Can you work these out from the model? Positions are in its coordinate system, mm. A direction names the side the tool comes from. Coordinates: 2 decimals unless noted, no trailing zeros. Order: outer loops, then holes, each group sorted by start corner. A loop starts at its lowest first (then second) coordinate and runs counter-clockwise, first axis right, second up. Notation, with made-up numbers: (50.5, 0.25) -> (57.5, 0.25) arc R25 cw to (57.5, 27.25) -> close; hole circle Ø5 at (78, 8.5). An arc over 180 degrees is marked (long way). Answer in a Markdown table with one row per item.
```python
from build123d import *

# Parameters (mm, degrees)
ESQUISSE1_R                  = 18.5
BOSS_EXTRU_1_DEPTH           = 30.7
ESQUISSE2_R                  = 5
BOSS_EXTRU_2_DEPTH           = 6
ESQUISSE3_R                  = 3
BOSS_EXTRU_3_DEPTH           = 16
ENL_V_MAT_EXTRU_2_DEPTH      = 59.836978168
ENL_V_MAT_EXTRU_2_DEPTH_BACK = 16


with BuildPart() as part:
    # Esquisse1 → Boss.-Extru.1 (new body)
    with BuildSketch(Plane.XY):
        Circle(ESQUISSE1_R)
    extrude(amount=BOSS_EXTRU_1_DEPTH)

    # Esquisse2 → Boss.-Extru.2 (add)
    with BuildSketch(Plane(origin=(0, 0, 0), x_dir=(-1, 0, 0), z_dir=(0, 0, -1))):
        Circle(ESQUISSE2_R)
    extrude(amount=BOSS_EXTRU_2_DEPTH)

    # Esquisse3 → Boss.-Extru.3 (add)
    with BuildSketch(Plane(origin=(0, 0, -6), x_dir=(-1, 0, 0), z_dir=(0, 0, -1))):
        Circle(ESQUISSE3_R)
    extrude(amount=BOSS_EXTRU_3_DEPTH)

    # Esquisse4 → Enlèv. mat.-Extru.2 (cut, two sides: drawn at the far end of the back side and taken through both)
    with BuildSketch(Plane(origin=(0, 0, -22), x_dir=(-1, 0, 0), z_dir=(0, 0, -1)).offset(-ENL_V_MAT_EXTRU_2_DEPTH_BACK)):
        Polygon((-70.071777045, 2.4), (-1.8, 2.4), (1.8, 2.4), (70.071777045, 2.4), (70.071777045, 138.94355409), (-70.071777045, 138.94355409), align=None)
    extrude(amount=ENL_V_MAT_EXTRU_2_DEPTH + ENL_V_MAT_EXTRU_2_DEPTH_BACK, mode=Mode.SUBTRACT)


solid = part.part
```
(1) Suppose I cut it at A-A (y = 0). Please give me the cut outline in (x, z).
Response values:
| item | result |
|---|---|
| outline | (-18.5, 0) -> (-5, 0) -> (-5, -6) -> (-3, -6) -> (-3, -22) -> (3, -22) -> (3, -6) -> (5, -6) -> (5, 0) -> (18.5, 0) -> (18.5, 30.7) -> (-18.5, 30.7) -> close |
(2) Suppose I cut it at D-D (z = -4). Please give me the cut outline in (x, y).
Response values:
| item | result |
|---|---|
| outline | circle Ø10 at (0, 0) |
(3) Suppose I cut it at C-C (z = -11). Please give me the cut outline in (x, y), and give its area (3 significant figures).
Response values:
| item | result |
|---|---|
| outline | (-1.8, 2.4) arc R3 ccw (long way) to (1.8, 2.4) -> close |
| area | 26.8 mm2 |
(4) Suppose I cut it at B-B (x = 0). Please give me the cut outline in (y, z), and give its area (3 significant figures).
Response values:
| item | result |
|---|---|
| outline | (-18.5, 0) -> (-5, 0) -> (-5, -6) -> (-3, -6) -> (-3, -22) -> (2.4, -22) -> (2.4, -6) -> (5, -6) -> (5, 0) -> (18.5, 0) -> (18.5, 30.7) -> (-18.5, 30.7) -> close |
| area | 1,280 mm2 |
(5) Will these pins go through, and if not, where does the flat tip stop? pin 1 Ø2 at (x, z) = (13, 25) entering from +Y; pin 2 Ø1.8 at (x, z) = (-0.5, -15) entering from +Y; pin 3 Ø12 at (y, z) = (-7.5, 5.5) entering from +X.
Response values:
| item | result |
|---|---|
| pin 1 | y = 14.08 |
| pin 2 | y = 2.4 |
| pin 3 | x = 18.44 |
(6) On a 3-axis mill with a long thin cutter (end or side, diameter ignored), from which of +Z, -Z, +X, -X, +Y, -Y can I reach the whole of each face in a straight line? I mean faces 1 (the cylindrical face through (0, -3, -14)), 2 (the flat face through (0, 2.4, -14)), 3 (the flat face through (0, 0, -22)). Say none if no direction works.
Response values:
| item | result |
|---|---|
| face 1 | -Z |
| face 2 | -Z, +X, -X, +Y |
| face 3 | -Z, +X, -X, +Y, -Y |
(7) I need wall thicknesses on line 1 (Z direction, x = 4, y = -4); line 2 (Z direction, x = -0.5, y = -3); line 3 (X direction, y = -2.5, z = -12). Which ranges of each line are inside material? Lowest first, please. Write a range as [from, to].
Response values:
| item | result |
|---|---|
| line 1 | [0, 30.7] |
| line 2 | [-6, 30.7] |
| line 3 | [-1.66, 1.66] |
